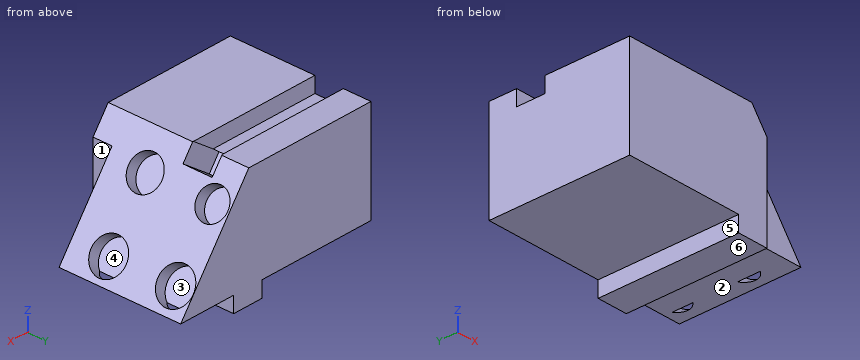
from build123d import *

# Parameters (mm, degrees)
F1_DEPTH  = 101.6
F2_W      = 95.392908901
F2_H      = 20.5622557551
F3_DEPTH  = 11.176
F5_W      = 21.0552625358
F5_H      = 13.1527595222
F6_DEPTH  = 25.4
F7_R      = 12.0900311227
F7_R_2    = 11.1649780349
F7_R_3    = 12.6885276411
F7_R_4    = 12.8258511979
F8_DEPTH  = 9.398
F10_DEPTH = 13.716


with BuildPart() as f1:
    # F0 (on Front) → F1 (new body)
    with BuildSketch(Plane.XZ):
        Polygon((32.0974774659, 39.2414145172), (-63.2954314351, 39.2414145172), (-63.2954314351, -33.8319987059), (21.8787807971, -33.8319987059), (21.8787807971, -45.1878346503), (43.9058281481, -45.1878346503), (43.9058281481, -33.8319987059), (85.2973610163, -33.8319987059), align=None)
    extrude(amount=F1_DEPTH)

    # F2 (on face) → F3 (cut)
    with BuildSketch(Plane.XY.offset(39.2414145172)):
        with Locations((-15.5989769846, -30.2323354408)):
            Rectangle(F2_W, F2_H)
    extrude(amount=-F3_DEPTH, mode=Mode.SUBTRACT)

    # F5 (on face) → F6 (cut)
    with BuildSketch(Plane(origin=(39.6504866209, 0, 28.8668775402), x_dir=(0, 1, 0), z_dir=(0.8084434725, 0, 0.5885738287))):
        with Locations((-30.0295893103, 6.5763797611)):
            Rectangle(F5_W, F5_H)
    extrude(amount=-F6_DEPTH, mode=Mode.SUBTRACT)

    # F7 (on face) → F8 (cut)
    with BuildSketch(Plane(origin=(39.6504866209, 0, 28.8668775402), x_dir=(0, 1, 0), z_dir=(0.8084434725, 0, 0.5885738287))):
        with Locations((-60.9646290541, -12.6676354557)):
            Circle(F7_R)
        with Locations((-12.3755605891, -12.6676354557)):
            Circle(F7_R_2)
        with Locations((-60.9646290541, -61.1499175429)):
            Circle(F7_R_3)
        with Locations((-13.0234146491, -60.3485517204)):
            Circle(F7_R_4)
    extrude(amount=-F8_DEPTH, mode=Mode.SUBTRACT)

    # F9 (on face) → F10 (cut)
    with BuildSketch(Plane.XZ.offset(101.6)):
        Polygon((43.9058281481, 31.8253524601), (43.9058281481, -33.8319987059), (85.2973610163, -33.8319987059), align=None)
    extrude(amount=-F10_DEPTH, mode=Mode.SUBTRACT)


solid = f1.part
Model file for the job. Use its own axes, mm. Face numbers are marked on the shaded views. A direction names the side the tool comes from. Give positions to 0.01 mm unless a question says otherwise; leave off trailing zeros. Loops run counter-clockwise (first coordinate to the right, second up) from the corner with the lowest first, then second, coordinate; pieces in that order, holes last. Notation, with made-up numbers: (75.5, -19) -> (90.5, -19) arc R12 ccw to (90.5, -14) -> close; hole circle Ø8 at (31, 29). An arc over 180 degrees is marked (long way). Use a Markdown table: item, result. Add a question column.
(1) Slice it at B-B on y = -58. List the corners of the cut face in (x, z).
(2) Slice it at C-C on x = 14. List the corners of the cut face in (y, z).
(3) Slice it at A-A on x = -36. List the corners of the cut face in (y, z).
(4) Wall check: line 1 along Y through (x, z) = (71.5, -23.5); line 2 along Y through (x, z) = (71, -17); line 3 along Z through (x, y) = (-12, -44). Give the ranges that are in metal, low to high.
(5) Drop flat-ended pins along their axis: pin 1 Ø5 at (x, y) = (55, -71.5) entering from -Z; pin 2 Ø3.5 at (y, z) = (-65, -42) entering from -X; pin 3 Ø20.5 at (x, z) = (67, -8) entering from -Y. Give the stop position or say it passes through.
(6) Mould opens along X. For the marked faces 4, 5 and 6 say: +X half, -X half, draft (parallel to the pull), parting line (faces both ways), or undercut.
(7) Tool access for the marked faces 1, 2 and 3: list every direction of +Z, -Z, +X, -X, +Y, -Y with a clear straight run to the whole face (end or side of a thin tool).
(8) Slice it at D-D on y = -14. List the corners of the cut face in (x, z).
Filled sheet:
| question | item | result |
|---|---|---|
| 1 | outline | (-63.3, -33.83) -> (21.88, -33.83) -> (21.88, -45.19) -> (43.91, -45.19) -> (43.91, -33.83) -> (73.67, -33.83) -> (60.78, -16.13) -> (68.38, -10.6) -> (54, 9.15) -> (46.41, 3.62) -> (32.61, 22.57) -> (40.21, 28.1) -> (32.1, 39.24) -> (-63.3, 39.24) -> close; (78.39, -33.83) -> (85.3, -33.83) -> (82.9, -30.54) -> close |
| 2 | outline | (-101.6, -33.83) -> (0, -33.83) -> (0, 39.24) -> (-19.95, 39.24) -> (-19.95, 28.07) -> (-40.51, 28.07) -> (-40.51, 39.24) -> (-101.6, 39.24) -> close; hole (-40.56, 20.94) -> (-19.5, 20.94) -> (-19.5, 26.46) -> (-40.56, 26.46) -> close |
| 3 | outline | (-101.6, -33.83) -> (0, -33.83) -> (0, 39.24) -> (-19.95, 39.24) -> (-19.95, 28.07) -> (-40.51, 28.07) -> (-40.51, 39.24) -> (-101.6, 39.24) -> close |
| 4 | line 1 | -87.88 to -73.65, -48.28 to -25.83, -0.22 to 0 |
| 4 | line 2 | -87.88 to -72.34, -49.59 to -24.91, -1.14 to 0 |
| 4 | line 3 | -33.83 to 39.24 |
| 5 | pin 1 | z = -33.83 |
| 5 | pin 2 | x = 21.88 |
| 5 | pin 3 | y = -87.88 |
| 6 | face 4 | undercut |
| 6 | face 5 | -X half |
| 6 | face 6 | draft |
| 7 | face 1 | -Z, +X, -Y |
| 7 | face 2 | -Z, +X, +Y, -Y |
| 7 | face 3 | none |
| 8 | outline | (-63.3, -33.83) -> (21.88, -33.83) -> (21.88, -45.19) -> (43.91, -45.19) -> (43.91, -33.83) -> (73.67, -33.83) -> (60.05, -15.11) -> (67.64, -9.58) -> (53.61, 9.7) -> (46.01, 4.16) -> (33.01, 22.02) -> (40.6, 27.56) -> (32.1, 39.24) -> (-63.3, 39.24) -> close; (77.79, -33.83) -> (85.3, -33.83) -> (82.7, -30.26) -> close |
